Work out the finished part from the listing and answer in its coordinate system (mm). Face numbers are marked on the shaded views. A direction names the side the tool comes from. Give positions to 0.01 mm unless a question says otherwise; leave off trailing zeros. Order: outer loops, then holes, each group sorted by start corner. A loop starts at its lowest first (then second) coordinate and runs counter-clockwise, first axis right, second up.
Autodesk Inventor part; units mm, degrees
ref_plane "YZ Plane" through (0, 0, 0) normal (1, 0, 0) x (0, 1, 0)
ref_plane "XZ Plane" through (0, 0, 0) normal (0, 1, 0) x (-1, 0, 0)
ref_plane "XY Plane" through (0, 0, 0) normal (0, 0, 1) x (1, 0, 0)
sketch "Sketch1" plane through (0, 0, 0) normal (0, 0, 1) x (1, 0, 0)
  line L0 (-23.3654, 0) -> (-10.6654, 0)
  line L1 (-10.6654, 0) -> (-10.6654, 121.92)
  line L2 (-10.6654, 121.92) -> (-23.3654, 121.92)
  line L3 (-23.3654, 121.92) -> (-23.3654, 0)
  circle A0 centre (-17.0154, 121.92) radius 38.1
  point P0 (0, 0)
  point P1 (-10.6654, 84.3529)
  point P2 (-23.3654, 84.3529)
  point P3 (-17.0154, 88.9)
  point P4 (-17.0154, 88.9)
  dimension "d1" = 76.2
  dimension "d2" = 121.92
  dimension "d4" = 12.7
  dimension "d5" = 6.35
revolve "Revolution5" add sketch "Sketch1" angle 360 about axis through (-23.3654, 0, 0) along (1, 0, 0)
sketch "Sketch3" plane through (-23.3654, 0, 0) normal (-1, 0, 0) x (0, 0, 1)
  circle A0 centre (0, 0) radius 19.05
  dimension "d10" = 38.1
extrude "Extrusion1" add sketch "Sketch3" along normal blind 25.4
sketch "Sketch4" plane through (-48.7654, 0, 0) normal (-1, 0, 0) x (0, 0, 1)
  circle A0 centre (0, 0) radius 11.1125
  dimension "d13" = 22.225
extrude "Extrusion2" cut sketch "Sketch4" against normal blind 25.4
sketch "Sketch5" plane through (-10.6654, 0, 0) normal (1, 0, 0) x (0, 0, -1)
  circle A0 centre (0, 0) radius 19.05
  circle A1 centre (0, 0) radius 16.891
  dimension "d16" = 38.1
  dimension "d17" = 33.782
extrude "Extrusion3" add sketch "Sketch5" along normal blind 47.625
sketch "Sketch6" plane through (-10.6654, 0, 0) normal (1, 0, 0) x (0, 0, -1)
  circle A0 centre (0, 0) radius 11.1125
  circle A1 centre (0, 0) radius 16.891
  point P0 (0, 0)
extrude "Extrusion4" cut sketch "Sketch6" against normal blind 76.2 contours A0 | A1
properties part number "Savior Wheel"
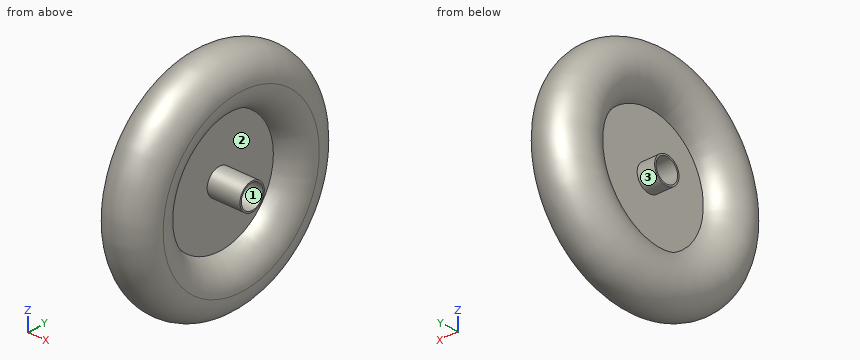
1. Which of the six approach directions +Z, -Z, +X, -X, +Y, -Y give full straight-line access (tool end or side, diameter ignored) to the marked faces 1, 2 and 3?
Findings below:
face 1: +X, -X
face 2: +X
face 3: -X
2. The part is cut by section C-C (x = 0.5). Write down the section's boundary in (y, z).
Findings below:
outline: circle Ø311.51 at (0, 0); circle Ø38.1 at (0, 0); hole circle Ø176.17 at (0, 0); hole circle Ø33.78 at (0, 0)
3. Straight lines are drawn through the part: probe 1 along Z at (x, y) = (-46, 12.5); probe 2 along X at (y, z) = (-80, 17); probe 3 along Z at (x, y) = (-35.5, -21). For each, find the intervals that lie inside material, in ascending order.
Findings below:
probe 1: z = -146.11 to -96.38, -14.38 to -11.36, 11.36 to 14.38, 96.38 to 146.11
probe 2: x = -23.37 to -10.67
probe 3: z = -153.81 to -86.08, 86.08 to 153.81
4. The part is cut by section A-A (y = 0). Write down the section's boundary in (x, z).
Findings below:
outline: (-48.77, -19.05) - (-23.37, -19.05) - (-23.37, -84.35) arc R38.1 ccw (long way) to (-10.67, -84.35) - (-10.67, -19.05) - (36.96, -19.05) - (36.96, -16.89) - (-48.77, -16.89) - close; (-48.77, 16.89) - (36.96, 16.89) - (36.96, 19.05) - (-10.67, 19.05) - (-10.67, 84.35) arc R38.1 ccw (long way) to (-23.37, 84.35) - (-23.37, 19.05) - (-48.77, 19.05) - close
5. Given P1, Ø1.5, axis at y = 42.5, z = 113, coming from the -X side; P2, Ø8, axis at x = -38, y = -54.5, coming from the -Z side; P3, Ø5, axis at x = -45, z = 8, coming from the -Y side, each flat-ended and moving along its own axis, determine where each tip first touches the part or whether it passes through.
Findings below:
P1: stops at x = -55.11
P2: stops at z = -146.64
P3: stops at y = -150.03
